CAD build for the part. Positions are in the model's coordinates, mm. Face numbers are marked on the shaded views. Round coordinates to 2 decimals unless told otherwise and drop trailing zeros. Order: outer loops, then holes, each group sorted by start corner. A loop starts at its lowest first (then second) coordinate and runs counter-clockwise, first axis right, second up.
```python
from build123d import *

# Parameters (mm, degrees)
F0_W     = 100
F0_H     = 50
F1_DEPTH = 5
F2_R     = 15
F3_DEPTH = 15
F4_R     = 4
F5_DEPTH = 20.001
F7_D     = 5.25
F8_R     = 2.15
F9_DEPTH = 25.001


with BuildPart() as f1:
    # F0 (on Top) → F1 (new body)
    with BuildSketch(Plane.XY):
        Rectangle(F0_W, F0_H)
    extrude(amount=F1_DEPTH)

    # F2 (on face) → F3 (join)
    with BuildSketch(Plane.XY.offset(5)):
        Circle(F2_R)
    extrude(amount=F3_DEPTH)

    # F4 (on face) → F5 (cut, through all)
    with BuildSketch(Plane.XY.offset(20)):
        Circle(F4_R)
    extrude(amount=-F5_DEPTH, mode=Mode.SUBTRACT)

    # F7 (through all)
    with Locations(Plane.XY.offset(5)):
        with Locations((-34.6410161514, 20), (-40, 0), (-34.6410161514, -20), (34.6410161514, 20), (40, 0), (34.6410161514, -20)):
            Hole(F7_D / 2)

    # F8 (on Front) → F9 (cut, through all)
    with BuildSketch(Plane.XZ):
        with Locations((0, 15)):
            Circle(F8_R)
    extrude(amount=-F9_DEPTH, mode=Mode.SUBTRACT)


solid = f1.part
```
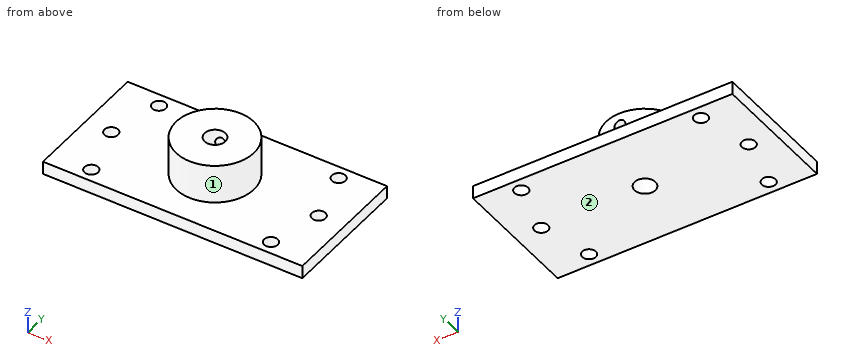
1. Drill centre lines: line 1 (Y direction, x = 40, z = 3.1) (3 decimals); line 2 (Z direction, x = -18, y = -3.5); line 3 (Y direction, x = -33.5, z = 2.25). Where is each one in solid material? Low to high.
2. Cut at A-A, the plane x = -40. Write the cut outline in (y, z) (3 decimals), and give its area (3 significant figures).
3. Mould opens along X. For the marked faces 1 and 2 say: released by +X, released by -X, zero draft, split by the parting line, or undercut.
4. Pin check, flat tips, straight feed: P1, Ø5.5, axis at x = 0, z = 15, coming from the +Y side; P2, Ø2, axis at y = 9, z = 7, coming from the -X side; P3, Ø1, axis at y = 13.5, z = 11.5, coming from the +X side. Stop position of each tip, or through.
5. Cut at C-C, the plane y = 0. Write the cut outline in (x, z) (3 decimals).
6. Cut at B-B, the plane z = 3. Write the cut outline in (x, y) (3 decimals).
7. Cut at D-D, the plane x = 0. Write the cut outline in (y, z), and give its area (3 significant figures).
Outcome:
1. line 1: y = -25 to -2.625, 2.625 to 25
1. line 2: z = 0 to 5
1. line 3: y = -25 to -22.36, -17.64 to 17.64, 22.36 to 25
2. outline: (-25, 0) - (-2.625, 0) - (-2.625, 5) - (-25, 5) - close; (2.625, 0) - (25, 0) - (25, 5) - (2.625, 5) - close
2. area: 224 mm2
3. face 1: split by the parting line
3. face 2: zero draft
4. P1: stops at y = 15
4. P2: stops at x = -12.69
4. P3: stops at x = 7.48
5. outline: (-50, 0) - (-42.625, 0) - (-42.625, 5) - (-50, 5) - close; (-37.375, 0) - (-4, 0) - (-4, 20) - (-15, 20) - (-15, 5) - (-37.375, 5) - close; (4, 0) - (37.375, 0) - (37.375, 5) - (15, 5) - (15, 20) - (4, 20) - close; (42.625, 0) - (50, 0) - (50, 5) - (42.625, 5) - close
6. outline: (-50, -25) - (50, -25) - (50, 25) - (-50, 25) - close; hole circle Ø5.25 at (-40, 0); hole circle Ø5.25 at (-34.641, -20); hole circle Ø5.25 at (-34.641, 20); hole circle Ø8 at (0, 0); hole circle Ø5.25 at (34.641, -20); hole circle Ø5.25 at (34.641, 20); hole circle Ø5.25 at (40, 0)
7. outline: (-25, 0) - (-4, 0) - (-4, 20) - (-15, 20) - (-15, 5) - (-25, 5) - close; (4, 0) - (25, 0) - (25, 5) - (15, 5) - (15, 12.85) - (4, 12.85) - close; (4, 17.15) - (15, 17.15) - (15, 20) - (4, 20) - close
7. area: 493 mm2
